```python
from build123d import *

# Parameters (mm, degrees)
SKETCH1_W               = 30
SKETCH1_H               = 25.4
BOSS_EXTRUDE1_DEPTH     = 8
CUT_EXTRUDE1_DEPTH      = 22.2200377
CUT_EXTRUDE1_DEPTH_BACK = 22.2200377
SKETCH2_R               = 4.45
SKETCH3_R               = 1.35
BOSS_EXTRUDE2_DEPTH     = 2
FILLET1_R               = 0.3
CHAMFER1_SIZE           = 0.2
SKETCH4_W               = 8
SKETCH4_H               = 12
CUT_EXTRUDE2_DEPTH      = 22.2200377
BOSS_EXTRUDE3_DEPTH     = 2
CHAMFER2_SIZE           = 1
FILLET2_R               = 0.5
CHAMFER3_SIZE           = 3
FILLET3_R               = 2


with BuildPart() as part:
    # Sketch1 → Boss-Extrude1 (new body)
    with BuildSketch(Plane.XY):
        Rectangle(SKETCH1_W, SKETCH1_H)
    extrude(amount=BOSS_EXTRUDE1_DEPTH)

    # Sketch2 → Cut-Extrude1 (cut, two sides: drawn at the far end of the back side and taken through both)
    with BuildSketch(Plane(origin=(0, 0, 0), x_dir=(1, 0, 0), z_dir=(0, 1, 0)).offset(-CUT_EXTRUDE1_DEPTH_BACK)):
        Circle(SKETCH2_R)
    extrude(amount=CUT_EXTRUDE1_DEPTH + CUT_EXTRUDE1_DEPTH_BACK, mode=Mode.SUBTRACT)

    # Sketch3 → Boss-Extrude2 (add)
    with BuildSketch(Plane.XY):
        with Locations((-12, 9.15)):
            Circle(SKETCH3_R)
        with Locations((12, 9.15)):
            Circle(SKETCH3_R)
        with Locations((12, -9.55)):
            Circle(SKETCH3_R)
        with Locations((-12, -9.55)):
            Circle(SKETCH3_R)
    extrude(amount=-BOSS_EXTRUDE2_DEPTH)

    # Fillet1
    fillet1_edges = [part.edges().sort_by_distance(p)[0] for p in [
        (-13.35, 9.15, 0),
        (10.65, 9.15, 0),
        (10.65, -9.55, 0),
        (-13.35, -9.55, 0),
    ]]
    fillet(fillet1_edges, radius=FILLET1_R)

    # Chamfer1
    chamfer1_edges = [part.edges().sort_by_distance(p)[0] for p in [
        (-13.35, 9.15, -2),
        (10.65, 9.15, -2),
        (10.65, -9.55, -2),
        (-13.35, -9.55, -2),
    ]]
    chamfer(chamfer1_edges, length=CHAMFER1_SIZE)

    # Sketch4 → Cut-Extrude2 (cut, through all)
    with BuildSketch(Plane.XY):
        with Locations((-11, -0.4)):
            Rectangle(SKETCH4_W, SKETCH4_H)
        with Locations((11, -0.4)):
            Rectangle(SKETCH4_W, SKETCH4_H)
    extrude(amount=CUT_EXTRUDE2_DEPTH, mode=Mode.SUBTRACT)

    # Sketch5 → Boss-Extrude3 (add, symmetric)
    with BuildSketch(Plane(origin=(0, 0, 0), x_dir=(0, 0, -1), z_dir=(1, 0, 0))):
        Polygon((-8, 5), (-8, -5), (-12.5, -3.5), (-12.5, -1.5), (-11, -1.5), (-11, -2.5), (-9, -2.5), (-9, 2.5), (-11, 2.5), (-11, 1.5), (-12.5, 1.5), (-12.5, 3.5), align=None)
    extrude(amount=BOSS_EXTRUDE3_DEPTH, both=True)

    # Chamfer2
    chamfer2_edges = [part.edges().sort_by_distance(p)[0] for p in [
        (2, 0, 8),
        (-2, 0, 8),
    ]]
    chamfer(chamfer2_edges, length=CHAMFER2_SIZE - 0.0001)  # a hair under: the kernel refuses the full size

    # Fillet2
    fillet2_edges = [part.edges().sort_by_distance(p)[0] for p in [
        (0, 3.5, 12.5),
        (0, 2.5, 11),
        (0, 2.5, 9),
        (0, -2.5, 9),
        (0, -2.5, 11),
        (0, -3.5, 12.5),
    ]]
    fillet(fillet2_edges, radius=FILLET2_R)

    # Chamfer3
    chamfer3_edges = [part.edges().sort_by_distance(p)[0] for p in [
        (-7, -0.4, 8),
        (7, -0.4, 8),
    ]]
    chamfer(chamfer3_edges, length=CHAMFER3_SIZE)

    # Fillet3
    fillet3_edges = [part.edges().sort_by_distance(p)[0] for p in [
        (-15, 9.15, 8),
        (15, -9.55, 8),
        (15, 9.15, 8),
        (-15, -9.55, 8),
    ]]
    fillet(fillet3_edges, radius=FILLET3_R)


solid = part.part
```
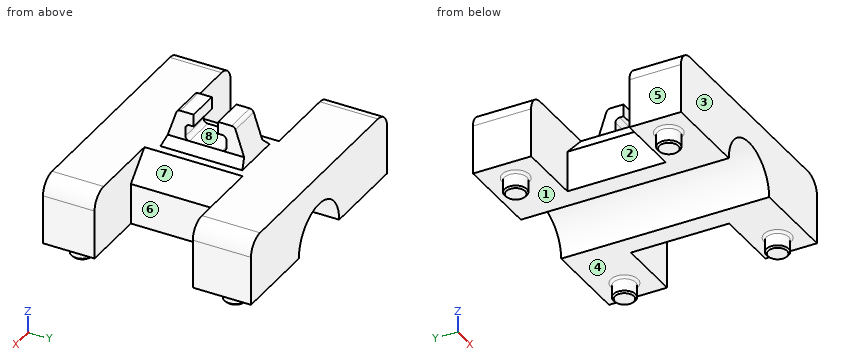
Build history of the part. All positions in model axes, mm. Face numbers are marked on the shaded views. A direction names the side the tool comes from. Coordinates: 2 decimals unless noted, no trailing zeros. Write each loop counter-clockwise with the first axis right and the second up, starting at its lowest first coordinate (ties: lowest second). Pieces come first, ordered by that corner, then holes.
1. Band-saw the part on A-A, the plane x = -8. Give the cut face in (y, z).
Answer block:
outline: (-12.7, 0) - (-6.4, 0) - (-6.4, 8) - (-12.7, 8) - close; (5.6, 0) - (12.7, 0) - (12.7, 8) - (5.6, 8) - close
2. 3-axis set-ups, long thin cutter, end or side, ignore diameter. For the marked faces 4, 5, 6, 7 and 8: which of +Z, -Z, +X, -X, +Y, -Y reach the whole face in a straight line?
Answer block:
face 4: -Z
face 5: +Z, -Z, -X, +Y, -Y
face 6: +Z, -Z, +X
face 7: +Z, +X
face 8: +X, -X
3. Drill centre lines: probe 1 along Y at (x, z) = (-9.5, 0.25); probe 2 along X at (y, z) = (-10.25, -0.25); probe 3 along Z at (x, y) = (4.75, -9). Where is each one in solid material? Low to high.
Answer block:
probe 1: y = -12.7 to -6.4, 5.6 to 12.7
probe 2: x = -13.16 to -10.84, 10.84 to 13.16
probe 3: z = 0 to 8
4. Drop flat-ended pins along their axis: pin 1 (5 mm diameter, centred on y = 2, z = 3, fed in from -X); pin 2 (6 mm diameter, centred on y = 1.5, z = 2, fed in from +X); pin 3 (4 mm diameter, centred on y = 1, z = 10.5, fed in from -X). Give the stop position or say it passes through.
Answer block:
pin 1: stops at x = -7
pin 2: stops at x = 7
pin 3: stops at x = -2.5
5. Pull direction X, two halves, no side cores. Call the marked faces 1, 2 and 3: released by +X, released by -X, zero draft, split by the parting line, or undercut.
Answer block:
face 1: undercut
face 2: released by -X
face 3: zero draft
6. Band-saw the part on D-D, the plane x = -12. Give the cut face in (y, z), and give its area (3 significant figures).
Answer block:
outline: (-12.7, 0) - (-11.2, 0) arc R0.3 cw to (-10.9, -0.3) - (-10.9, -1.8) - (-10.7, -2) - (-8.4, -2) - (-8.2, -1.8) - (-8.2, -0.3) arc R0.3 cw to (-7.9, 0) - (-6.4, 0) - (-6.4, 8) - (-12.7, 8) - close; (5.6, 0) - (7.5, 0) arc R0.3 cw to (7.8, -0.3) - (7.8, -1.8) - (8, -2) - (10.3, -2) - (10.5, -1.8) - (10.5, -0.3) arc R0.3 cw to (10.8, 0) - (12.7, 0) - (12.7, 8) - (5.6, 8) - close
area: 118 mm2
7. Band-saw the part on B-B, the plane z = 3. Give the cut face in (x, y).
Answer block:
outline: (-15, -12.7) - (-3.29, -12.7) - (-3.29, 12.7) - (-15, 12.7) - (-15, 5.6) - (-7, 5.6) - (-7, -6.4) - (-15, -6.4) - close; (3.29, -12.7) - (15, -12.7) - (15, -6.4) - (7, -6.4) - (7, 5.6) - (15, 5.6) - (15, 12.7) - (3.29, 12.7) - close
8. Band-saw the part on C-C, the plane y = 9.15. Give the cut face in (x, z), and give its area (3 significant figures).
Answer block:
outline: (-15, 0) - (-13.65, 0) arc R0.3 cw to (-13.35, -0.3) - (-13.35, -1.8) - (-13.15, -2) - (-10.85, -2) - (-10.65, -1.8) - (-10.65, -0.3) arc R0.3 cw to (-10.35, 0) - (-4.45, 0) arc R4.45 cw to (4.45, 0) - (10.35, 0) arc R0.3 cw to (10.65, -0.3) - (10.65, -1.8) - (10.85, -2) - (13.15, -2) - (13.35, -1.8) - (13.35, -0.3) arc R0.3 cw to (13.65, 0) - (15, 0) - (15, 6) arc R2 ccw to (13, 8) - (-13, 8) arc R2 ccw to (-15, 6) - close
area: 218 mm2
